For this review, take the finished solid that the model builds, in its own axes (mm). Face numbers are marked on the shaded views. A direction names the side the tool comes from. Coordinates: 2 decimals unless noted, no trailing zeros. Write each loop counter-clockwise with the first axis right and the second up, starting at its lowest first coordinate (ties: lowest second). Pieces come first, ordered by that corner, then holes. Notation, with made-up numbers: (86.25, 75) - (109.25, 75) arc R26 ccw to (109.25, 94) - close; hole circle Ø4 at (59, -7). An arc over 180 degrees is marked (long way). Use one line per item in the form item = value. Start each with the question number.
1) For L1, parallel to Y at x = 0.95, z = 0.2; L2, parallel to X at y = 5.5, z = 0.15; L3, parallel to Z at x = 0, y = 3, list the stretches that pass through material, from the lowest coordinate up. Write a range as from..to.
2) We need section A-A (y = 5). Give the boundary of the cut face in (x, z), plus the area to 3 significant figures.
3) Insertion check: P1, Ø0.5, axis at y = 5.5, z = -1, coming from the +X side; P2, Ø2, axis at y = 3.5, z = -2, coming from the +X side; P3, Ø0.5, axis at x = 0.5, y = 5.5, coming from the +Z side. Each pin has a flat end and moves straight along its axis. Give the tip position at first contact, or say it passes through.
4) We need section B-B (y = 1.75). Give the boundary of the cut face in (x, z).
5) Tool access review of the marked faces 1 and 2: name each direction out of +Z, -Z, +X, -X, +Y, -Y from which nothing blocks a thin tool from reaching the whole face with its end or side.
6) Mouldability with a two-part tool opening along X and no side actions: class the marked faces 3, 4 and 5 as pulls with the +X half, pulls with the -X half, needs draft (parallel to the pull), parting line crosses it, or undercut.
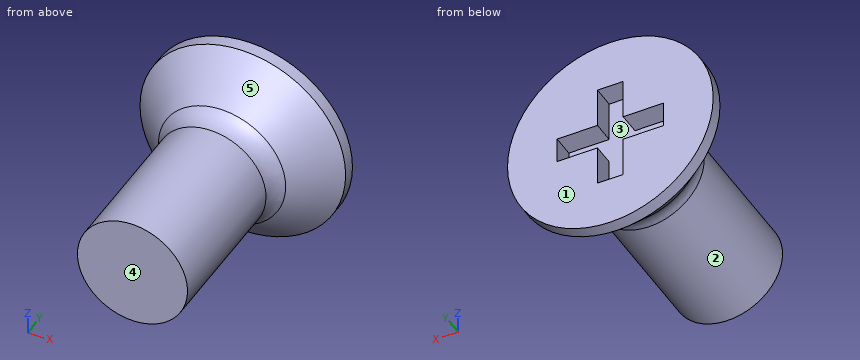
```python
from build123d import *

# Parameters (mm, degrees)
FILLET1_R          = 0.8
SKETCH2_W          = 1.1
SKETCH2_H          = 0.7
SKETCH2_W_2        = 0.7
SKETCH2_H_2        = 1.1
CUT_EXTRUDE1_DEPTH = 0.6


with BuildPart() as part:
    # Sketch1 → Revolve1 (revolve)
    with BuildSketch(Plane.XY):
        Polygon((0, 0), (0, 6), (2.8, 6), (2.8, 5.65), (1.5, 4.35), (1.5, 0), align=None)
    revolve(axis=Axis((0, 0, 0), (0, 1, 0)))

    # Fillet1
    fillet1_edges = [part.edges().sort_by_distance(p)[0] for p in [
        (-1.5, 4.35, 0),
    ]]
    fillet(fillet1_edges, radius=FILLET1_R)

    # Sketch2 → Cut-Extrude1 (cut)
    with BuildSketch(Plane(origin=(0, 6, 0), x_dir=(1, 0, 0), z_dir=(0, 1, 0))):
        with Locations((-0.9, 0)):
            Rectangle(SKETCH2_W, SKETCH2_H)
        with Locations((0, 0.9)):
            Rectangle(SKETCH2_W_2, SKETCH2_H_2)
        Rectangle(SKETCH2_W_2, SKETCH2_H)
        with Locations((0.9, 0)):
            Rectangle(SKETCH2_W, SKETCH2_H)
        with Locations((0, -0.9)):
            Rectangle(SKETCH2_W_2, SKETCH2_H_2)
    extrude(amount=-CUT_EXTRUDE1_DEPTH, mode=Mode.SUBTRACT)


solid = part.part
```
Determined:
q1.L1 = 0..5.4
q1.L2 = -2.65..-1.45, 1.45..2.65
q1.L3 = -1.5..1.5
q2.outline = circle Ø4.3 at (0, 0)
q2.area = 14.5 mm²
q3.P1 = 2.68
q3.P2 = 1.12
q3.P3 = 2.78
q4.outline = circle Ø3 at (0, 0)
q5.face_1 = +Z, -Z, +X, -X, +Y
q5.face_2 = -Y
q6.face_3 = undercut
q6.face_4 = needs draft
q6.face_5 = parting line crosses it
